Verification items for the finished model (mm, model axes). A direction names the side the tool comes from. Round coordinates to 2 decimals unless told otherwise and drop trailing zeros. Write each loop counter-clockwise with the first axis right and the second up, starting at its lowest first coordinate (ties: lowest second). Pieces come first, ordered by that corner, then holes. Notation, with made-up numbers: M -35,24 L -26,24 A27 ccw -26,62 Z; hole C 26.5,-1.5 d2. An arc over 180 degrees is marked long. Write each question's results on one line, items separated by ' | '.
from build123d import *

# Parameters (mm, degrees)
BOSS_EXTRUDE1_DEPTH = 5
SKETCH4_W           = 3.75
SKETCH4_H           = 2.5
CUT_EXTRUDE2_DEPTH  = 101
SKETCH5_R           = 0.36
CUT_EXTRUDE3_DEPTH  = 81
FILLET1_R           = 1.2
FILLET2_R           = 1.2


with BuildPart() as part:
    # Sketch1 → Boss-Extrude1 (new body)
    with BuildSketch(Plane.XY):
        Polygon((0, 0), (0, 100), (5, 100), (5, 5), (55, 5), (55, 100), (60, 100), (60, 50), (60, 32), (80, 32), (80, 0), align=None)
    extrude(amount=BOSS_EXTRUDE1_DEPTH)

    # Sketch4 → Cut-Extrude2 (cut, through all)
    with BuildSketch(Plane(origin=(0, 100, 0), x_dir=(1, 0, 0), z_dir=(0, 1, 0))):
        with Locations((56.875, -2.5)):
            Rectangle(SKETCH4_W, SKETCH4_H)
        with Locations((3.125, -2.5)):
            Rectangle(SKETCH4_W, SKETCH4_H)
    extrude(amount=-CUT_EXTRUDE2_DEPTH, mode=Mode.SUBTRACT)

    # Sketch5 → Cut-Extrude3 (cut, through all)
    with BuildSketch(Plane(origin=(80, 0, 0), x_dir=(0, 0, -1), z_dir=(1, 0, 0))):
        with Locations((-2.5, 25)):
            Circle(SKETCH5_R)
    extrude(amount=-CUT_EXTRUDE3_DEPTH, mode=Mode.SUBTRACT)

    # Fillet1
    fillet1_edges = [part.edges().sort_by_distance(p)[0] for p in [
        (40, 0, 0),
    ]]
    fillet(fillet1_edges, radius=FILLET1_R)

    # Fillet2
    fillet2_edges = [part.edges().sort_by_distance(p)[0] for p in [
        (40, 0, 5),
    ]]
    fillet(fillet2_edges, radius=FILLET2_R)


solid = part.part
1) Draft check along Z on faces 1 (the flat face through (0, 49, 2)), 2 (the flat face through (58, 33, 0)), 3 (the flat face through (57, 51, 1.25)). Enter one of: pulls with the +Z half, pulls with the -Z half, needs draft (parallel to the pull), parting line crosses it, or undercut.
Calculated:
face 1: needs draft | face 2: pulls with the -Z half | face 3: undercut
2) Sectioned sample at B-B, the plane x = 71. Record the cut outline in (y, z), and give its area (3 significant figures).
Calculated:
outline: M 0,1.2 A1.2 ccw 1.2,0 L 32,0 L 32,5 L 1.2,5 A1.2 ccw 0,3.8 Z; hole C 25,2.5 d0.72 | area: 159 mm²
3) Access from +Z, -Z, +X, -X, +Y, -Y to the whole of each face (thin tool, end or side, straight path). Record for faces 4 (the flat face through (30, 5, 2)), 5 (the flat face through (70, 32, 2)), 6 (the flat face through (59, 100, 2)), 7 (the flat face through (1.25, 51, 3)).
Calculated:
face 4: +Z, -Z, +Y | face 5: +Z, -Z, +X, +Y | face 6: +Z, -Z, +X, -X, +Y | face 7: +Y, -Y
4) Sectioned sample at C-C, the plane y = 19. Record the cut outline in (x, z), and give its area (3 significant figures).
Calculated:
outline: M 0,0 L 5,0 L 5,1.25 L 1.25,1.25 L 1.25,3.75 L 5,3.75 L 5,5 L 0,5 Z; M 55,0 L 80,0 L 80,5 L 55,5 L 55,3.75 L 58.75,3.75 L 58.75,1.25 L 55,1.25 Z | area: 131 mm²
5) Depth check by flat-ended pin: P1, Ø0.8, axis at y = 3, z = 3, coming from the -X side; P2, Ø1, axis at y = 50.5, z = 0.5, coming from the +X side. Enter the tip coordinate at first touch or a pass-through.
Calculated:
P1: stops at x = 0 | P2: stops at x = 60
6) Sectioned sample at D-D, the plane x = 27. Record the cut outline in (y, z), and give its area (3 significant figures).
Calculated:
outline: M 0,1.2 A1.2 ccw 1.2,0 L 5,0 L 5,5 L 1.2,5 A1.2 ccw 0,3.8 Z | area: 24.4 mm²
7) Sectioned sample at A-A, the plane y = 58.5. Record the cut outline in (x, z), and give its area (4 significant figures).
Calculated:
outline: M 0,0 L 5,0 L 5,1.25 L 1.25,1.25 L 1.25,3.75 L 5,3.75 L 5,5 L 0,5 Z; M 55,0 L 60,0 L 60,5 L 55,5 L 55,3.75 L 58.75,3.75 L 58.75,1.25 L 55,1.25 Z | area: 31.25 mm²
8) Material ranges on line 1 (X direction, y = 92.5, z = 4.6); line 2 (X direction, y = 6, z = 2.5); line 3 (Z direction, x = 64, y = 25), recorded low to high. Write a range as [from, to].
Calculated:
line 1: x = [0, 5], [55, 60] | line 2: x = [0, 1.25], [58.75, 80] | line 3: z = [0, 2.14], [2.86, 5]
